from build123d import *

# Parameters (mm, degrees)
BOX_W           = 10
BOX_H           = 10
BOX_DEPTH       = 10
POCKET_DEPTH    = 0.1
POCKET001_DEPTH = 0.1
POCKET002_DEPTH = 0.1
SKETCH003_W     = 9.983458
SKETCH003_H     = 1.354645
SKETCH003_W_2   = 9.983948
SKETCH003_W_3   = 4.247611
POCKET003_DEPTH = 0.1
SKETCH005_R     = 2.993458
POCKET004_DEPTH = 1
SKETCH004_R     = 3.024316
PAD_DEPTH       = 1.2
CHAMFER_SIZE    = 0.5


with BuildPart() as part:
    # Box → Box (new body)
    with BuildSketch(Plane.XY):
        with Locations((5, 5)):
            Rectangle(BOX_W, BOX_H)
    extrude(amount=BOX_DEPTH)

    # Sketch → Pocket (cut)
    with BuildSketch(Plane.XZ):
        Polygon((-0.013318, 2.848971), (-0.013318, -0.000633), (1.358424, -0.000633), align=None)
        Polygon((10.018128, 2.842927), (10.018128, -0.006678), (8.646385, -0.006678), align=None)
        Polygon((0.052197, 7.646552), (0.052197, 4.796948), (2.377994, -0.034572), (3.749737, -0.034572), align=None)
        Polygon((6.233827, 0), (7.605569, 0), (9.971137, 4.914136), (9.971137, 7.76374), align=None)
        Polygon((3.436299, 3.149153), (4.952238, 0), (6.468178, 3.149153), align=None)
        Polygon((2.093005, 5.965705), (2.8215, 4.452359), (7.216569, 4.452359), (7.945064, 5.965705), align=None)
        Polygon((0.513832, 8.838719), (1.242326, 7.325373), (8.661189, 7.325373), (9.389684, 8.838719), align=None)
    extrude(amount=-POCKET_DEPTH, mode=Mode.SUBTRACT)

    # Sketch001 → Pocket001 (cut)
    with BuildSketch(Plane(origin=(0, 0, 0), x_dir=(0, -1, 0), z_dir=(-1, 0, 0))):
        Polygon((-8.576619, 0), (-7.121317, 0), (-7.121317, 2.835466), (-9.956783, 2.835466), (-9.956783, 1.380163), (-8.576619, 1.380163), align=None)
        Polygon((-9.957004, 5.599077), (-9.957004, 4.143775), (-5.813229, 4.143775), (-5.813229, 0), (-4.357927, 0), (-4.357927, 5.599077), align=None)
        Polygon((-9.988727, 8.658869), (-9.988727, 7.203567), (-2.78516, 7.203567), (-2.78516, 0), (-1.329858, 0), (-1.329858, 8.658869), align=None)
    extrude(amount=-POCKET001_DEPTH, mode=Mode.SUBTRACT)

    # Sketch002 → Pocket002 (cut)
    with BuildSketch(Plane.YZ.offset(10)):
        Polygon((8.742587, 0), (8.742587, 1.482263), (9.971997, 1.482263), (9.971997, 2.769174), (7.455676, 2.769174), (7.455676, 0), align=None)
        Polygon((5.758296, 0), (5.758296, 4.296487), (9.989896, 4.296487), (9.989896, 5.583398), (4.471385, 5.583398), (4.471385, 0), align=None)
        Polygon((2.82081, 0), (2.82081, 7.153826), (9.974636, 7.153826), (9.974636, 8.440737), (1.533899, 8.440737), (1.533899, 0), align=None)
    extrude(amount=-POCKET002_DEPTH, mode=Mode.SUBTRACT)

    # Sketch003 → Pocket003 (cut)
    with BuildSketch(Plane(origin=(0, 10, 0), x_dir=(-1, 0, 0), z_dir=(0, 1, 0))):
        with Locations((-4.991729, 2.135502)):
            Rectangle(SKETCH003_W, SKETCH003_H)
        with Locations((-4.991974, 4.899971)):
            Rectangle(SKETCH003_W_2, SKETCH003_H)
        with Locations((-7.864695, 7.76353)):
            Rectangle(SKETCH003_W_3, SKETCH003_H)
        with Locations((-2.145795, 7.795235)):
            Rectangle(SKETCH003_W_3, SKETCH003_H)
    extrude(amount=-POCKET003_DEPTH, mode=Mode.SUBTRACT)

    # Sketch005 → Pocket004 (cut)
    with BuildSketch(Plane.XY.offset(10)):
        with Locations((4.99216, 5.03797)):
            Circle(SKETCH005_R)
    extrude(amount=-POCKET004_DEPTH, mode=Mode.SUBTRACT)

    # Sketch004 → Pad (new body)
    with BuildSketch(Plane(origin=(0, 0, 0), x_dir=(1, 0, 0), z_dir=(0, 0, -1))):
        with Locations((5.026122, -5.03797)):
            Circle(SKETCH004_R)
    extrude(amount=PAD_DEPTH)

    # Chamfer
    chamfer_edges = [part.edges().sort_by_distance(p)[0] for p in [
        (2.001806, 5.03797, -1.2),
    ]]
    chamfer(chamfer_edges, length=CHAMFER_SIZE)


solid = part.part
Check sheet for the modelled part. Datum: model origin and axes. Units: mm. A direction names the side the tool comes from. Give positions to 0.01 mm unless a question says otherwise; leave off trailing zeros. Loops run counter-clockwise (first coordinate to the right, second up) from the corner with the lowest first, then second, coordinate; pieces in that order, holes last. Notation, with made-up numbers: M -6.5,-6 L 25.5,-6 A21 ccw 25.5,6 Z; hole C 23.25,-9.5 d5. An arc over 180 degrees is marked long. Use a Markdown table: item, result. Add a question column.
Q1. Sectioned sample at C-C, the plane z = 9.25. Record the cut outline in (x, y).
Q2. Tool access check on faces 1 (the cylindrical face through (6.37, 2.38, 9.51)), 2 (the flat face through (1.5, 0.1, 3.3)), 3 (the flat face through (0.4, 0.1, 0.8)), 4 (the flat face through (9.6, 0.1, 0.8)). Record the directions out of +Z, -Z, +X, -X, +Y, -Y that give a thin tool (end or side, any length) a straight path to the whole face; none if there is none.
Q3. Go/stop test with a flat-tipped pin: pin 1 (1 mm diameter, centred on x = 1, y = 3, fed in from -Z). Record where the tip stops, or that it passes through.
Q4. Scan lines: line 1 along X through (y, z) = (8.5, 2); line 2 along Z through (x, y) = (1.75, 2.5); line 3 along Z through (x, y) = (3, 6.25). Record each from-to range of solid material in increasing order. Write a range as [from, to].
Q5. Mould release check, pull along X, two halves, no side actions. Record for faces 5 (the cylindrical face through (7.82, 6.2, -0.35)), 6 (the flat face through (5, 5, 9)), 7 (the flat face through (5, 0, 7)): pulls with the +X half, pulls with the -X half, needs draft (parallel to the pull), parting line crosses it, or undercut.
Q6. Sectioned sample at A-A, the plane z = 8. Give the number of separate pieces and of enclosed holes in the cut face, then the cut area to 3 significant figures.
Q7. Sectioned sample at B-B, the plane x = 9. Record the cut outline in (y, z), then the cut area to 3 significant figures.
Verdict:
| question | item | result |
|---|---|---|
| 1 | outline | M 0,0 L 10,0 L 10,10 L 0,10 Z; hole C 4.99,5.04 d5.99 |
| 2 | face 1 | +Z |
| 2 | face 2 | -Y |
| 2 | face 3 | -Z, -X, -Y |
| 2 | face 4 | -Z, +X, -Y |
| 3 | pin 1 | z = 0 |
| 4 | line 1 | [0.1, 9.9] |
| 4 | line 2 | [0, 10] |
| 4 | line 3 | [-1.2, 9] |
| 5 | face 5 | parting line crosses it |
| 5 | face 6 | undercut |
| 5 | face 7 | needs draft |
| 6 | separate pieces | 3 |
| 6 | enclosed holes | 0 |
| 6 | area | 96.6 mm^2 |
| 7 | outline | M 0,0.73 L 0.1,0.73 L 0.1,0 L 10,0 L 10,1.46 L 9.9,1.46 L 9.9,2.81 L 10,2.81 L 10,4.22 L 9.9,4.22 L 9.9,5.58 L 10,5.58 L 10,7.09 L 9.9,7.09 L 9.9,8.44 L 10,8.44 L 10,10 L 0,10 L 0,8.84 L 0.1,8.84 L 0.1,8.03 L 0,8.03 L 0,5.75 L 0.1,5.75 L 0.1,2.9 L 0,2.9 Z |
| 7 | area | 99.2 mm^2 |
